Could you check a few things on this model? Use its own coordinates, in mm. Face numbers are marked on the shaded views. Give positions to 0.01 mm unless a question says otherwise; leave off trailing zeros.
(1) Will these pins go through, and if not, where does the flat tip stop? pin 1 (2 mm diameter, centred on x = 2.5, z = 5.5, fed in from +Y); pin 2 (2 mm diameter, centred on x = 3, z = 5, fed in from -Y); pin 3 (2 mm diameter, centred on x = 2.5, z = 7, fed in from +Y).
(2) Imagine slicing it at C-C, the plane z = 4. State how many separate pieces and enclosed holes the cut face has, then the cut area to 3 significant figures.
(3) If we mould it in two halves opening along X, with no side actions, what happens to the marked faces 1, 2 and 3? For each: released by +X, released by -X, zero draft, split by the parting line, or undercut.
(4) If I drill on probe 1 along X at (y, z) = (4, 1.5); probe 2 along Y at (x, z) = (-8, 6.25); probe 3 along X at (y, z) = (-9.5, 5.25), over which ranges is the centre line in solid material (lowest first)?
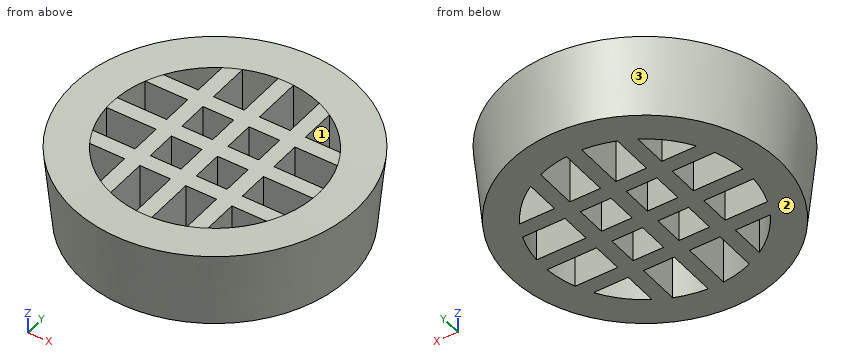
from build123d import *

# Parameters (mm, degrees)
F2_W     = 4
F2_H     = 4
F3_DEPTH = 10


with BuildPart() as f1:
    # F0 (on Front) → F1 (revolve)
    with BuildSketch(Plane.XZ):
        Polygon((-18.5, 10.194688), (-17.5, 0), (-13.5, 0), (-13.5, 10), align=None)
    revolve(axis=Axis((0, 0, 3.021993), (0, 0, -1)))

    # F2 (on Top) → F3 (join)
    with BuildSketch(Plane.XY):
        with BuildLine():
            Line((-7, 7), (-11.666143, 7))
            ThreePointArc((-11.666143, 7), (-12.200632, 6.020256), (-12.653019, 5))
            Line((-12.653019, 5), (-7, 5))
            Line((-7, 5), (-7, 1))
            Line((-7, 1), (-13.568305, 1))
            ThreePointArc((-13.568305, 1), (-13.605106, 0), (-13.568305, -1))
            Line((-13.568305, -1), (-7, -1))
            Line((-7, -1), (-7, -5))
            Line((-7, -5), (-12.653019, -5))
            ThreePointArc((-12.653019, -5), (-12.200632, -6.020256), (-11.666143, -7))
            Line((-11.666143, -7), (-7, -7))
            Line((-7, -7), (-7, -11.666143))
            ThreePointArc((-7, -11.666143), (-6.020256, -12.200632), (-5, -12.653019))
            Line((-5, -12.653019), (-5, -7))
            Line((-5, -7), (-1, -7))
            Line((-1, -7), (-1, -13.568305))
            ThreePointArc((-1, -13.568305), (0, -13.605106), (1, -13.568305))
            Line((1, -13.568305), (1, -7))
            Line((1, -7), (5, -7))
            Line((5, -7), (5, -12.653019))
            ThreePointArc((5, -12.653019), (6.020256, -12.200632), (7, -11.666143))
            Line((7, -11.666143), (7, -7))
            Line((7, -7), (11.666143, -7))
            ThreePointArc((11.666143, -7), (12.200632, -6.020256), (12.653019, -5))
            Line((12.653019, -5), (7, -5))
            Line((7, -5), (7, -1))
            Line((7, -1), (13.568305, -1))
            ThreePointArc((13.568305, -1), (13.605106, 0), (13.568305, 1))
            Line((13.568305, 1), (7, 1))
            Line((7, 1), (7, 5))
            Line((7, 5), (12.653019, 5))
            ThreePointArc((12.653019, 5), (12.200632, 6.020256), (11.666143, 7))
            Line((11.666143, 7), (7, 7))
            Line((7, 7), (7, 11.666143))
            ThreePointArc((7, 11.666143), (6.020256, 12.200632), (5, 12.653019))
            Line((5, 12.653019), (5, 7))
            Line((5, 7), (1, 7))
            Line((1, 7), (1, 13.568305))
            ThreePointArc((1, 13.568305), (0, 13.605106), (-1, 13.568305))
            Line((-1, 13.568305), (-1, 7))
            Line((-1, 7), (-5, 7))
            Line((-5, 7), (-5, 12.653019))
            ThreePointArc((-5, 12.653019), (-6.020256, 12.200632), (-7, 11.666143))
            Line((-7, 11.666143), (-7, 7))
        make_face()
        with Locations((-3, -3)):
            Rectangle(F2_W, F2_H, mode=Mode.SUBTRACT)
        with Locations((3, -3)):
            Rectangle(F2_W, F2_H, mode=Mode.SUBTRACT)
        with Locations((-3, 3)):
            Rectangle(F2_W, F2_H, mode=Mode.SUBTRACT)
        with Locations((3, 3)):
            Rectangle(F2_W, F2_H, mode=Mode.SUBTRACT)
    extrude(amount=F3_DEPTH)


solid = f1.part
Answer block:
1. pin 1: stops at y = 18.02
1. pin 2: stops at y = -17.91
1. pin 3: stops at y = 18.17
2. separate pieces: 1
2. enclosed holes: 16
2. area: 698 mm2
3. face 1: undercut
3. face 2: zero draft
3. face 3: split by the parting line
4. probe 1: x = -17.19 to -12.89, -7 to -5, -1 to 1, 5 to 7, 12.89 to 17.19
4. probe 2: y = -16.25 to -10.87, -7 to -5, -1 to 1, 5 to 7, 10.87 to 16.25
4. probe 3: x = -15.31 to -9.59, -7 to -5, -1 to 1, 5 to 7, 9.59 to 15.31
